Build history of the part. All positions in model axes, mm. A direction names the side the tool comes from. Give positions to 0.01 mm unless a question says otherwise; leave off trailing zeros. Loops run counter-clockwise (first coordinate to the right, second up) from the corner with the lowest first, then second, coordinate; pieces in that order, holes last. Notation, with made-up numbers: (-7, 81.25) -> (28, 81.25) arc R22 ccw to (28, 118.25) -> close; hole circle Ø9 at (19.25, 52). An arc over 180 degrees is marked (long way). Answer in a Markdown table with one row per item. Add a question column.
from build123d import *

# Parameters (mm, degrees)
BOSS_EXTRUDE1_DEPTH = 100
SKETCH2_W           = 35
SKETCH2_H           = 30
CUT_EXTRUDE1_DEPTH  = 139.001578957
SKETCH3_W           = 20
SKETCH3_H           = 15
BOSS_EXTRUDE2_DEPTH = 10
SKETCH4_W           = 20
SKETCH4_H           = 15
BOSS_EXTRUDE3_DEPTH = 10
BOSS_EXTRUDE4_DEPTH = 15
CUT_EXTRUDE2_DEPTH  = 134.603892159


with BuildPart() as part:
    # Sketch1 → Boss-Extrude1 (new body)
    with BuildSketch(Plane.XY):
        with BuildLine():
            Line((0, 0), (0, 12.701945525))
            Line((0, 12.701945525), (40, 12.701945525))
            Line((40, 12.701945525), (40, 27.701945525))
            Line((40, 27.701945525), (20, 27.701945525))
            ThreePointArc((20, 27.701945525), (12.928932188, 30.630877713), (10, 37.701945525))
            Line((10, 37.701945525), (10, 52.701945525))
            Line((10, 52.701945525), (15, 52.701945525))
            Line((15, 52.701945525), (15, 67.701945525))
            Line((15, 67.701945525), (10, 67.701945525))
            Line((10, 67.701945525), (10, 82.701945525))
            ThreePointArc((10, 82.701945525), (-31.652166191, 45.782811211), (0, 0))
        make_face()
    extrude(amount=BOSS_EXTRUDE1_DEPTH)

    # Sketch2 → Cut-Extrude1 (cut, through all)
    with BuildSketch(Plane(origin=(15, 0, 0), x_dir=(0, 0, -1), z_dir=(1, 0, 0))):
        with Locations((-52.5, 67.701945525)):
            Rectangle(SKETCH2_W, SKETCH2_H)
    extrude(amount=-CUT_EXTRUDE1_DEPTH, mode=Mode.SUBTRACT)

    # Sketch3 → Boss-Extrude2 (add)
    with BuildSketch(Plane.XY.offset(100)):
        with Locations((5, 60.201945525)):
            Rectangle(SKETCH3_W, SKETCH3_H)
    extrude(amount=BOSS_EXTRUDE2_DEPTH)

    # Sketch4 → Boss-Extrude3 (add)
    with BuildSketch(Plane(origin=(0, 0, 0), x_dir=(-1, 0, 0), z_dir=(0, 0, -1))):
        with Locations((-5, 60.201945525)):
            Rectangle(SKETCH4_W, SKETCH4_H)
    extrude(amount=BOSS_EXTRUDE3_DEPTH)

    # Sketch5 → Boss-Extrude4 (add)
    with BuildSketch(Plane.XY.offset(100)):
        with BuildLine():
            Line((40, 17.701945525), (-31.20321015, 32.836655055))
            ThreePointArc((-31.20321015, 32.836655055), (-20.413872841, 11.845443896), (0, 0))
            Line((0, 0), (0, 12.701945525))
            Line((0, 12.701945525), (40, 12.701945525))
            Line((40, 12.701945525), (40, 17.701945525))
        make_face()
    extrude(amount=BOSS_EXTRUDE4_DEPTH)

    # Sketch6 → Cut-Extrude2 (cut, through all)
    with BuildSketch(Plane(origin=(0, 27.701945525, 0), x_dir=(1, 0, 0), z_dir=(0, 1, 0))):
        with BuildLine():
            Line((35, -10), (35, -90))
            ThreePointArc((35, -90), (30, -95), (25, -90))
            Line((25, -90), (25, -10))
            ThreePointArc((25, -10), (30, -5), (35, -10))
        make_face()
    extrude(amount=-CUT_EXTRUDE2_DEPTH, mode=Mode.SUBTRACT)


solid = part.part
(1) Saw through at B-B, the plane y = 69.5. List the corners of the cut face in (x, z), then the cut area to 3 significant figures.
(2) Flat gauge pins, fed straight in: pin 1 Ø16.5 at (y, z) = (45.5, 37.5) entering from +X; pin 2 Ø9 at (x, y) = (-18.5, 71) entering from -Z; pin 3 Ø10 at (x, z) = (-13, 51.5) entering from +Y. Where does each tip first touch, or does it go through?
(3) Wall check: line 1 along Y through (x, z) = (-12, 43); line 2 along Z through (x, y) = (4.5, 46); line 3 along Z through (x, y) = (28.5, 22). Give the ranges that are in metal, low to high. Write a range as from..to.
(4) Saw through at D-D, the plane x = -25. List the corners of the cut face in (y, z).
(5) Two-plate mould, pull along Y, no slides. Class faces 6 (the flat face through (10, 45, 49)), 7 (the flat face through (20, 12.702, 57)), 8 (the flat face through (35, 20, 49)): released by +Y, released by -Y, zero draft, split by the parting line, or undercut.
(6) Saw through at A-A, the plane z = 15.5. List the corners of the cut face in (x, y).
(7) Saw through at C-C, the plane x = 30. List the corners of the cut face in (y, z).
(8) 3-axis set-ups, long thin cutter, end or side, ignore diameter. For faces 1 (the flat face through (-5, 60, 105)), 2 (the flat face through (4.897, 25.163, 107.395)), 3 (the flat face through (5, 60, 110)), 4 (the cylindrical face through (30, 20, 95)), 5 (the flat face through (15, 60, 13)): which of +Z, -Z, +X, -X, +Y, -Y reach the whole face in a straight line?
Worked answers:
| question | item | result |
|---|---|---|
| 1 | outline | (-20.55, 0) -> (10, 0) -> (10, 35) -> (-20.55, 35) -> close; (-20.55, 70) -> (10, 70) -> (10, 100) -> (-20.55, 100) -> close |
| 1 | area | 1,990 mm^2 |
| 2 | pin 1 | x = 15 |
| 2 | pin 2 | z = 0 |
| 2 | pin 3 | y = 52.7 |
| 3 | line 1 | 5.02..52.7 |
| 3 | line 2 | 0..100 |
| 3 | line 3 | 0..5.23, 94.77..100 |
| 4 | outline | (17.61, 0) -> (63.88, 0) -> (63.88, 35) -> (52.7, 35) -> (52.7, 70) -> (63.88, 70) -> (63.88, 100) -> (31.52, 100) -> (31.52, 115) -> (17.61, 115) -> close |
| 5 | face 6 | undercut |
| 5 | face 7 | released by -Y |
| 5 | face 8 | zero draft |
| 6 | outline | (0, 0) -> (0, 12.7) -> (25, 12.7) -> (25, 27.7) -> (20, 27.7) arc R10 cw to (10, 37.7) -> (10, 52.7) -> (15, 52.7) -> (15, 67.7) -> (10, 67.7) -> (10, 82.7) arc R41.96 ccw to start; (35, 12.7) -> (40, 12.7) -> (40, 27.7) -> (35, 27.7) -> close |
| 7 | outline | (12.7, 0) -> (27.7, 0) -> (27.7, 5) -> (12.7, 5) -> close; (12.7, 95) -> (27.7, 95) -> (27.7, 100) -> (19.83, 100) -> (19.83, 115) -> (12.7, 115) -> close |
| 8 | face 1 | +Z, -X, +Y |
| 8 | face 2 | +Z, +X |
| 8 | face 3 | +Z, +X, -X, +Y |
| 8 | face 4 | +Y, -Y |
| 8 | face 5 | +Z, -Z, +X, +Y |
